Source: CAD feature listing. Evaluate the final solid. Frame: model axes, mm. A direction names the side the tool comes from. Give positions to 0.01 mm unless a question says otherwise; leave off trailing zeros. Loops run counter-clockwise (first coordinate to the right, second up) from the corner with the lowest first, then second, coordinate; pieces in that order, holes last. Notation, with made-up numbers: M 0,9 L 9,9 A32 cw 9,45 Z; hole C 9,5.5 d7. An arc over 180 degrees is marked long. Write item = value, one per line.
from build123d import *

# Parameters (mm, degrees)
SKETCH1_W           = 135
SKETCH1_H           = 122
BOSS_EXTRUDE1_DEPTH = 5.7
CUT_EXTRUDE1_DEPTH  = 6
HOLE_W              = 50
HOLE_H              = 80
CUT_EXTRUDE2_DEPTH  = 70
SCREW_LOCATIONS_R   = 1
CUT_EXTRUDE3_DEPTH  = 52


with BuildPart() as part:
    # Sketch1 → Boss-Extrude1 (new body)
    with BuildSketch(Plane(origin=(0, 0, 0), x_dir=(0, 0, -1), z_dir=(1, 0, 0))):
        with Locations((67.5, 61)):
            Rectangle(SKETCH1_W, SKETCH1_H)
    extrude(amount=BOSS_EXTRUDE1_DEPTH)

    # Sketch2 → Cut-Extrude1 (cut)
    with BuildSketch(Plane(origin=(0, 0, 0), x_dir=(0, 0, -1), z_dir=(1, 0, 0))):
        Polygon((0, 116), (27, 116), (27, 121.7), (54, 121.7), (54, 116), (81, 116), (81, 121.7), (108, 121.7), (108, 116), (135, 116), (135, 130), (0, 130), align=None)
        Polygon((0, -8), (0, 6), (27, 6), (27, 0.3), (54, 0.3), (54, 6), (81, 6), (81, 0.3), (108, 0.3), (108, 6), (135, 6), (135, -8), align=None)
    extrude(amount=CUT_EXTRUDE1_DEPTH, mode=Mode.SUBTRACT)

    # Hole → Cut-Extrude2 (cut)
    with BuildSketch(Plane(origin=(0, 0, 0), x_dir=(0, 0, -1), z_dir=(1, 0, 0))):
        with Locations((55, 60)):
            Rectangle(HOLE_W, HOLE_H)
    extrude(amount=CUT_EXTRUDE2_DEPTH, mode=Mode.SUBTRACT)

    # Screw Locations → Cut-Extrude3 (cut)
    with BuildSketch(Plane(origin=(0, 0, 0), x_dir=(0, 0, -1), z_dir=(1, 0, 0))):
        with Locations((25.23, 104.17)):
            Circle(SCREW_LOCATIONS_R)
        with Locations((84.77, 104.17)):
            Circle(SCREW_LOCATIONS_R)
        with Locations((25.23, 15.83)):
            Circle(SCREW_LOCATIONS_R)
        with Locations((84.77, 15.83)):
            Circle(SCREW_LOCATIONS_R)
    extrude(amount=CUT_EXTRUDE3_DEPTH, mode=Mode.SUBTRACT)


solid = part.part
1. Reachability of faces 1 (the flat face through (3, 119, -108)), 2 (the flat face through (3, 3, -27)), 3 (the flat face through (3, 3, -108)) from +Z, -Z, +X, -X, +Y, -Y: full face, straight path, thin tool, end or side. Return the list, or none.
Derived:
face_1 = -Z, +X, -X, +Y
face_2 = +Z, +X, -X, -Y
face_3 = -Z, +X, -X, -Y
2. Cut plane C-C, the plane x = 1.1. Return the cut outline in (y, z), then the cut area to 3 significant figures.
Derived:
outline = M 0.3,-108 L 6,-108 L 6,-135 L 116,-135 L 116,-108 L 121.7,-108 L 121.7,-81 L 116,-81 L 116,-54 L 121.7,-54 L 121.7,-27 L 116,-27 L 116,0 L 6,0 L 6,-27 L 0.3,-27 L 0.3,-54 L 6,-54 L 6,-81 L 0.3,-81 Z; hole C 15.83,-84.77 d2; hole C 15.83,-25.23 d2; hole M 20,-80 L 100,-80 L 100,-30 L 20,-30 Z; hole C 104.17,-84.77 d2; hole C 104.17,-25.23 d2
area = 11,500 mm²
3. First-contact query: pin 1 Ø1.7 at (x, z) = (4, -127.5) entering from +Y. Flat tip, straight axial feed; report the tip coordinate or a pass-through.
Derived:
pin_1 = 116
4. Cut plane B-B, the plane y = 25.5. Return the cut outline in (x, z).
Derived:
outline = M 0,-135 L 5.7,-135 L 5.7,-80 L 0,-80 Z; M 0,-30 L 5.7,-30 L 5.7,0 L 0,0 Z
5. Cut plane A-A, the plane z = -42. Return the cut outline in (x, y).
Derived:
outline = M 0,0.3 L 5.7,0.3 L 5.7,20 L 0,20 Z; M 0,100 L 5.7,100 L 5.7,121.7 L 0,121.7 Z
6. Material intervals for probe 1 along Y at (x, z) = (1.3, -25.23); probe 2 along Y at (x, z) = (3.8, -84.77); probe 3 along Z at (x, y) = (4, 15.83), sorted ascending. Write a range as from..to.
Derived:
probe_1 = 6..14.83, 16.83..103.17, 105.17..116
probe_2 = 0.3..14.83, 16.83..103.17, 105.17..121.7
probe_3 = -135..-85.77, -83.77..-26.23, -24.23..0
7. Pull-direction query (Y, two-part tool) for faces 4 (the flat face through (3, 60, -135)), 5 (the flat face through (3, 6, -121)), 6 (the flat face through (3, 20, -55)); classes: +Y half, -Y half, draft (parallel to the pull), parting line (faces both ways), or undercut.
Derived:
face_4 = draft
face_5 = -Y half
face_6 = undercut
